Input: dimensioned drawing with shaded views. Units: mm. Origin: part minimum x, y, z. A direction names the side the tool comes from. Coordinates: 2 decimals unless noted, no trailing zeros. Write each loop counter-clockwise with the first axis right and the second up, starting at its lowest first coordinate (ties: lowest second). Pieces come first, ordered by that corner, then holes. Notation, with made-up numbers: M 0,-32.5 L 18,-32.5 A12 cw 18,-25.5 Z; hole C -19,65 d2. An arc over 180 degrees is marked long. Use one line per item in the form item = value.
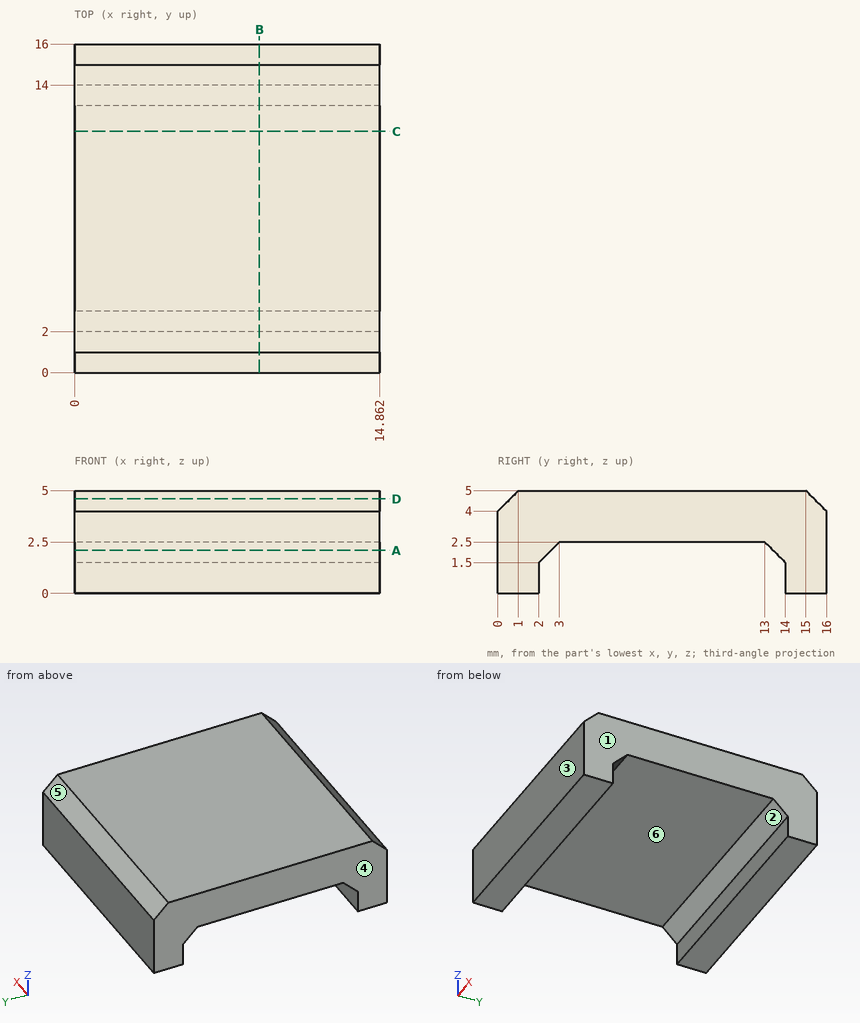
(1) Section query D-D on z = 4.6. Return the cut outline in (x, y), plus the area to 3 significant figures.
Computed:
outline = M 0,0.6 L 14.86,0.6 L 14.86,15.4 L 0,15.4 Z
area = 220 mm^2
(2) Set-up query: the marked faces 1 and 2. Return all of +Z, -Z, +X, -X, +Y, -Y with unobstructed straight access to the full face (end or side cutting, diameter ignored); none if empty.
Computed:
face_1 = +Z, -Z, +X, +Y, -Y
face_2 = -Z, +X, -X
(3) First-contact query: pin 1 Ø1.5 at (y, z) = (11.5, 3) entering from -X. Flat tip, straight axial feed; report the tip coordinate or a pass-through.
Computed:
pin_1 = 0
(4) Section query A-A on z = 2.1. Return the cut outline in (x, y).
Computed:
outline = M 0,0 L 14.86,0 L 14.86,2.6 L 0,2.6 Z; M 0,13.4 L 14.86,13.4 L 14.86,16 L 0,16 Z
(5) Line query: probe 1 along Y at (x, z) = (8.25, 0.35); probe 2 along Z at (x, y) = (9.5, 7); probe 3 along Y at (x, z) = (10, 2.2). Output: solid intervals per line, ascending.
Computed:
probe_1 = 0 to 2, 14 to 16
probe_2 = 2.5 to 5
probe_3 = 0 to 2.7, 13.3 to 16
(6) Section query B-B on x = 9. Return the cut outline in (y, z).
Computed:
outline = M 0,0 L 2,0 L 2,1.5 L 3,2.5 L 13,2.5 L 14,1.5 L 14,0 L 16,0 L 16,4 L 15,5 L 1,5 L 0,4 Z
(7) Section query C-C on y = 11.75. Return the cut outline in (x, z).
Computed:
outline = M 0,2.5 L 14.86,2.5 L 14.86,5 L 0,5 Z
(8) Pull-direction query (Y, two-part tool) for the marked faces 3, 4, 5 and 6; classes: pulls with the +Y half, pulls with the -Y half, needs draft (parallel to the pull), parting line crosses it, or undercut.
Computed:
face_3 = pulls with the -Y half
face_4 = needs draft
face_5 = pulls with the +Y half
face_6 = undercut
